```python
from build123d import *

# Parameters (mm, degrees)
SKETCH1_W           = 558.8
SKETCH1_H           = 330.2
BOSS_EXTRUDE1_DEPTH = 12.7
SKETCH4_R           = 9.525
CUT_EXTRUDE1_DEPTH  = 12.7


with BuildPart() as part:
    # Sketch1 → Boss-Extrude1 (new body)
    with BuildSketch(Plane.XY):
        with Locations((279.4, -165.1)):
            Rectangle(SKETCH1_W, SKETCH1_H)
    extrude(amount=BOSS_EXTRUDE1_DEPTH)

    # Sketch4 → Cut-Extrude1 (cut)
    with BuildSketch(Plane(origin=(0, 0, 0), x_dir=(-1, 0, 0), z_dir=(0, 0, -1))):
        with Locations((-279.4, -304.8)):
            Circle(SKETCH4_R)
        with Locations((-524.764, -228.6)):
            Circle(SKETCH4_R)
        with Locations((-524.764, -127)):
            Circle(SKETCH4_R)
        with Locations((-34.036, -228.6)):
            Circle(SKETCH4_R)
        with Locations((-34.036, -127)):
            Circle(SKETCH4_R)
        with Locations((-524.764, -50.8)):
            Circle(SKETCH4_R)
        with Locations((-34.036, -50.8)):
            Circle(SKETCH4_R)
    extrude(amount=-CUT_EXTRUDE1_DEPTH, mode=Mode.SUBTRACT)


solid = part.part
```
CAD build for the part. Positions are in the model's coordinates, mm. Round coordinates to 2 decimals unless told otherwise and drop trailing zeros. Order: outer loops, then holes, each group sorted by start corner. A loop starts at its lowest first (then second) coordinate and runs counter-clockwise, first axis right, second up. Notation, with made-up numbers: (-8, 67.5) -> (10, 67.5) arc R29 ccw to (10, 91.5) -> close; hole circle Ø9 at (77.25, -33). An arc over 180 degrees is marked (long way). Write item = value, one per line.
(1) Cut at A-A (y = -304.8). Write the cut outline in (x, z) (3 decimals), plus the area to 3 significant figures.
Answers follow:
outline = (0, 0) -> (269.875, 0) -> (269.875, 12.7) -> (0, 12.7) -> close; (288.925, 0) -> (558.8, 0) -> (558.8, 12.7) -> (288.925, 12.7) -> close
area = 6,850 mm²
(2) Pull direction Y, two halves, no side cores. Call faces 1 (the flat face through (558.8, -167, 6)), 2 (the flat face through (275, 0, 6)), 3 (the cylindrical face through (41.056, -44.363, 6.261)): +Y half, -Y half, draft (parallel to the pull), parting line (faces both ways), or undercut.
Answers follow:
face_1 = draft
face_2 = +Y half
face_3 = undercut
(3) Drill centre lines: L1, parallel to X at y = -121.5, z = 11.25; L2, parallel to X at y = -311.5, z = 6.75; L3, parallel to Y at x = 271.5, z = 10. Where is each one in solid material? Low to high.
Answers follow:
L1 = 0 to 26.26, 41.81 to 516.99, 532.54 to 558.8
L2 = 0 to 272.63, 286.17 to 558.8
L3 = -330.2 to -310.12, -299.48 to 0
(4) Cut at B-B (y = -50.8). Write the cut outline in (x, z), plus the area to 3 significant figures.
Answers follow:
outline = (0, 0) -> (24.51, 0) -> (24.51, 12.7) -> (0, 12.7) -> close; (43.56, 0) -> (515.24, 0) -> (515.24, 12.7) -> (43.56, 12.7) -> close; (534.29, 0) -> (558.8, 0) -> (558.8, 12.7) -> (534.29, 12.7) -> close
area = 6,610 mm²
